```python
from build123d import *

# Parameters (mm, degrees)
SKETCH1_W            = 11
SKETCH1_H            = 22
BOSS_EXTRUDE1_DEPTH  = 17.5
SKETCH8_W            = 7
SKETCH8_H            = 4
BOSS_EXTRUDE6_DEPTH  = 7
FILLET1_R            = 1
FILLET2_R            = 1
SKETCH9_W            = 11
SKETCH9_H            = 2.5
BOSS_EXTRUDE7_DEPTH  = 4.5
SKETCH10_W           = 11
SKETCH10_H           = 2.5
BOSS_EXTRUDE8_DEPTH  = 4.5
CUT_EXTRUDE1_DEPTH   = 5
SKETCH2_R            = 4
BOSS_EXTRUDE9_DEPTH  = 8
SKETCH13_R           = 9.5
BOSS_EXTRUDE10_DEPTH = 2


with BuildPart() as part:
    # Sketch1 → Boss-Extrude1 (new body)
    with BuildSketch(Plane(origin=(0, 0, 0), x_dir=(1, 0, 0), z_dir=(0, 1, 0))):
        Rectangle(SKETCH1_W, SKETCH1_H)
    extrude(amount=BOSS_EXTRUDE1_DEPTH)

    # Sketch8 → Boss-Extrude6 (add)
    with BuildSketch(Plane.XY.offset(11)):
        with Locations((0, 2)):
            Rectangle(SKETCH8_W, SKETCH8_H)
    extrude(amount=BOSS_EXTRUDE6_DEPTH)

    # Fillet1
    fillet1_edges = [part.edges().sort_by_distance(p)[0] for p in [
        (-3.5, 0, 14.5),
        (-3.5, 4, 14.5),
        (3.5, 4, 14.5),
        (3.5, 0, 14.5),
    ]]
    fillet(fillet1_edges, radius=FILLET1_R)

    # Fillet2
    fillet2_edges = [part.edges().sort_by_distance(p)[0] for p in [
        (0, 0, 18),
        (-3.5, 2, 18),
        (3.5, 2, 18),
        (0, 4, 18),
        (3.207106781, 0.292893219, 18),
        (3.207106781, 3.707106781, 18),
        (-3.207106781, 3.707106781, 18),
        (-3.207106781, 0.292893219, 18),
    ]]
    fillet(fillet2_edges, radius=FILLET2_R)

    # Sketch9 → Boss-Extrude7 (add)
    with BuildSketch(Plane.XY.offset(11)):
        with Locations((0, 14.25)):
            Rectangle(SKETCH9_W, SKETCH9_H)
    extrude(amount=BOSS_EXTRUDE7_DEPTH)

    # Sketch10 → Boss-Extrude8 (add)
    with BuildSketch(Plane(origin=(0, 0, -11), x_dir=(-1, 0, 0), z_dir=(0, 0, -1))):
        with Locations((0, 14.25)):
            Rectangle(SKETCH10_W, SKETCH10_H)
    extrude(amount=BOSS_EXTRUDE8_DEPTH)

    # Sketch11 → Cut-Extrude1 (cut)
    with BuildSketch(Plane(origin=(0, 17.5, 0), x_dir=(1, 0, 0), z_dir=(0, 1, 0))):
        with BuildLine():
            Line((1.4, 15.5), (1.4, 14.928285686))
            ThreePointArc((1.4, 14.928285686), (0, 11.5), (-1.4, 14.928285686))
            Line((-1.4, 14.928285686), (-1.4, 15.5))
            Line((-1.4, 15.5), (1.4, 15.5))
        make_face()
        with BuildLine():
            Line((-1.4, -15.5), (-1.4, -14.928285686))
            ThreePointArc((-1.4, -14.928285686), (0, -11.5), (1.4, -14.928285686))
            Line((1.4, -14.928285686), (1.4, -15.5))
            Line((1.4, -15.5), (-1.4, -15.5))
        make_face()
    extrude(amount=-CUT_EXTRUDE1_DEPTH, mode=Mode.SUBTRACT)

    # Sketch2 → Boss-Extrude9 (add)
    with BuildSketch(Plane(origin=(0, 17.5, 0), x_dir=(1, 0, 0), z_dir=(0, 1, 0))):
        with Locations((0, -5.38022134)):
            Circle(SKETCH2_R)
    extrude(amount=BOSS_EXTRUDE9_DEPTH)

    # Sketch13 → Boss-Extrude10 (add)
    with BuildSketch(Plane(origin=(0, 25.5, 0), x_dir=(1, 0, 0), z_dir=(0, 1, 0))):
        with Locations((0, -5.38022134)):
            Circle(SKETCH13_R)
    extrude(amount=BOSS_EXTRUDE10_DEPTH)


solid = part.part
```
Source: CAD feature listing. Evaluate the final solid. Frame: model axes, mm. A direction names the side the tool comes from. Give positions to 0.01 mm unless a question says otherwise; leave off trailing zeros. Loops run counter-clockwise (first coordinate to the right, second up) from the corner with the lowest first, then second, coordinate; pieces in that order, holes last. Notation, with made-up numbers: (60.5, 89.5) -> (76.5, 89.5) arc R18 ccw to (76.5, 103.5) -> close; hole circle Ø8 at (-17.5, 33.25). An arc over 180 degrees is marked (long way). Put each result on its own line as item: value. Start each with the question number.
1) Cut plane D-D (z = 13.5). Return loops of the section in (x, y).
2) Cut plane B-B (y = 2.5). Return loops of the section in (x, z), then the cut area to 3 significant figures.
3) Reachability of faces 1 (the face through (0, 16, 11)), 2 (the face through (-3.199, 0.285, 14.042)), 3 (the face through (-0.07, 14.27, 11.5)), 4 (the face through (3, 14, 15.5)) from +Z, -Z, +X, -X, +Y, -Y: full face, straight path, thin tool, end or side. Return the list, or none.
4) Contact query for flat-ended pins moving along their axis: P1, Ø14, axis at y = 6, z = -2.5, coming from the +X side; P2, Ø4, axis at x = 5.5, y = 15, coming from the +Z side; P3, Ø2, axis at x = -1.5, y = 4.5, coming from the -Z side. Output: stop coordinate, or through.
5) Material intervals for probe 1 along Y at (x, z) = (2.5, 13); probe 2 along X at (y, z) = (14.2, 13.5); probe 3 along Z at (x, y) = (-2.25, 13.5), sorted ascending.
6) Cut plane A-A (z = -13.5). Return loops of the section in (x, y).
7) Cut plane C-C (x = 0). Return loops of the section in (y, z), then the cut area to 3 significant figures.
8) Draft query along Y for faces 5 (the face through (-3.5, 2, 14)), 6 (the face through (-0.035, 3.699, 17.715)), 7 (the face through (3.199, 3.715, 14.042)), 8 (the face through (-3.215, 3.699, 14.042)). Return one class per face: released by +Y, released by -Y, zero draft, split by the parting line, or undercut.
Results are:
1. outline: (-5.5, 13) -> (-2, 13) -> (-2, 15.5) -> (-5.5, 15.5) -> close; (-4.93, 25.5) -> (4.93, 25.5) -> (4.93, 27.5) -> (-4.93, 27.5) -> close; (-3.5, 1) arc R1 ccw to (-2.5, 0) -> (2.5, 0) arc R1 ccw to (3.5, 1) -> (3.5, 3) arc R1 ccw to (2.5, 4) -> (-2.5, 4) arc R1 ccw to (-3.5, 3) -> close; (2, 13) -> (5.5, 13) -> (5.5, 15.5) -> (2, 15.5) -> close
2. outline: (-5.5, -11) -> (5.5, -11) -> (5.5, 11) -> (3.5, 11) -> (3.5, 17) arc R1 ccw to (2.5, 18) -> (-2.5, 18) arc R1 ccw to (-3.5, 17) -> (-3.5, 11) -> (-5.5, 11) -> close
2. area: 291 mm2
3. face 1: +Z, +X, -X
3. face 2: +Z, -X, -Y
3. face 3: none
3. face 4: +Z, +X, -X, +Y
4. P1: stops at x = 5.5
4. P2: stops at z = 15.5
4. P3: stops at z = -11
5. probe 1: y = 0 to 4, 13 to 15.5, 25.5 to 27.5
5. probe 2: x = -5.5 to -2, 2 to 5.5
5. probe 3: z = -15.5 to 15.5
6. outline: (-5.5, 13) -> (-2, 13) -> (-2, 15.5) -> (-5.5, 15.5) -> close; (2, 13) -> (5.5, 13) -> (5.5, 15.5) -> (2, 15.5) -> close
7. outline: (0, -11) -> (13, -11) -> (13, -11.5) -> (15.5, -11.5) -> (15.5, -11) -> (17.5, -11) -> (17.5, 1.38) -> (25.5, 1.38) -> (25.5, -4.12) -> (27.5, -4.12) -> (27.5, 14.88) -> (25.5, 14.88) -> (25.5, 9.38) -> (17.5, 9.38) -> (17.5, 11) -> (15.5, 11) -> (15.5, 11.5) -> (13, 11.5) -> (13, 11) -> (4, 11) -> (4, 17) arc R1 ccw to (3, 18) -> (1, 18) arc R1 ccw to (0, 17) -> close
7. area: 517 mm2
8. face 5: zero draft
8. face 6: released by +Y
8. face 7: undercut
8. face 8: undercut
